Verification items for the finished model (mm, model axes). A direction names the side the tool comes from. Give positions to 0.01 mm unless a question says otherwise; leave off trailing zeros. Order: outer loops, then holes, each group sorted by start corner. A loop starts at its lowest first (then second) coordinate and runs counter-clockwise, first axis right, second up. Notation, with made-up numbers: (88, 75.25) -> (138, 75.25) arc R24 cw to (138, 110.25) -> close; hole circle Ø10 at (29.25, 45). An arc over 180 degrees is marked (long way). One line per question, with ' | ' between items. Start each with the question number.
Q1. Section check D-D on x = -28. Record the cut outline in (y, z), plus the area to 3 significant figures.
Q2. Mould release check, pull along X, two halves, no side actions. Record for faces 1 (the flat face through (123, 4, 4)), 2 (the cylindrical face through (1.609, 12.502, 4.437)), 3 (the flat face through (-123, 5, 4)), 4 (the flat face through (-2, 10, 9)): released by +X, released by -X, zero draft, split by the parting line, or undercut.
Q3. Section check C-C on x = 99. Record the cut outline in (y, z), plus the area to 3 significant figures.
Q4. Access from +Z, -Z, +X, -X, +Y, -Y to the whole of each face (thin tool, end or side, straight path). Record for faces 5 (the flat face through (-114, 13, 4)), 6 (the flat face through (114, 13, 4)), 7 (the flat face through (-2, 10, 0)).
Q5. Go/stop test with flat-tipped pins: pin 1 (2 mm diameter, centred on y = 11, z = 4, fed in from -X); pin 2 (1.5 mm diameter, centred on y = 14, z = 2, fed in from +X); pin 3 (2 mm diameter, centred on x = -50.5, z = 3.5, fed in from +Y). Record where each tip stops, or that it passes through.
Q6. Material ranges on probe 1 along X at (y, z) = (11.25, 2.5); probe 2 along Y at (x, z) = (-15, 2.5); probe 3 along Y at (x, z) = (-68, 3), recorded low to high. Write a range as [from, to].
Q7. Section check A-A on y = 15. Record the cut outline in (x, z).
Q8. Section check B-B on z = 5. Record the cut outline in (x, y), plus the area to 3 significant figures.
from build123d import *

# Parameters (mm, degrees)
BOSS_EXTRUDE2_DEPTH = 9
SKETCH2_W           = 9
SKETCH2_H           = 9
CUT_EXTRUDE1_DEPTH  = 126.837196409


with BuildPart() as part:
    # Sketch1 → Boss-Extrude2 (new body)
    with BuildSketch(Plane.XY):
        with BuildLine():
            Line((-123, 25), (-123, 0))
            Line((-123, 0), (123, 0))
            Line((123, 0), (123, 25))
            Line((123, 25), (114, 25))
            ThreePointArc((114, 25), (0, 12.5), (-114, 25))
            Line((-114, 25), (-123, 25))
        make_face()
    extrude(amount=BOSS_EXTRUDE2_DEPTH)

    # Sketch2 → Cut-Extrude1 (cut, through all)
    with BuildSketch(Plane.XY):
        with Locations((118.5, 13.5)):
            Rectangle(SKETCH2_W, SKETCH2_H)
        with Locations((-118.5, 13.5)):
            Rectangle(SKETCH2_W, SKETCH2_H)
    extrude(amount=CUT_EXTRUDE1_DEPTH, mode=Mode.SUBTRACT)


solid = part.part
Filled in:
1) outline: (0, 0) -> (13.25, 0) -> (13.25, 9) -> (0, 9) -> close | area: 119 mm²
2) face 1: released by +X | face 2: undercut | face 3: released by -X | face 4: zero draft
3) outline: (0, 0) -> (21.9, 0) -> (21.9, 9) -> (0, 9) -> close | area: 197 mm²
4) face 5: +Z, -Z, -X | face 6: +Z, -Z, +X | face 7: -Z, +X, -X, +Y, -Y
5) pin 1: x = -114 | pin 2: x = 114 | pin 3: y = 15.03
6) probe 1: [-114, 114] | probe 2: [0, 12.71] | probe 3: [0, 16.91]
7) outline: (-114, 0) -> (-51.23, 0) -> (-51.23, 9) -> (-114, 9) -> close; (51.23, 0) -> (114, 0) -> (114, 9) -> (51.23, 9) -> close
8) outline: (-123, 0) -> (123, 0) -> (123, 9) -> (114, 9) -> (114, 18) -> (123, 18) -> (123, 25) -> (114, 25) arc R526.09 cw to (-114, 25) -> (-123, 25) -> (-123, 18) -> (-114, 18) -> (-114, 9) -> (-123, 9) -> close | area: 4,080 mm²
